Work out the finished part from the listing and answer in its coordinate system (mm). A direction names the side the tool comes from. Coordinates: 2 decimals unless noted, no trailing zeros. Order: outer loops, then holes, each group sorted by start corner. A loop starts at its lowest first (then second) coordinate and runs counter-clockwise, first axis right, second up.
```python
from build123d import *

# Parameters (mm, degrees)
SKETCH1_R           = 133
BOSS_EXTRUDE1_DEPTH = 53.5
SKETCH2_R           = 125
BOSS_EXTRUDE2_DEPTH = 51
SKETCH3_R           = 100
BOSS_EXTRUDE3_DEPTH = 5
SKETCH4_R           = 106
BOSS_EXTRUDE4_DEPTH = 12
SKETCH5_R           = 60
BOSS_EXTRUDE5_DEPTH = 11
SKETCH6_R           = 35
CUT_EXTRUDE1_DEPTH  = 231.074444474


with BuildPart() as part:
    # Sketch1 → Boss-Extrude1 (new body)
    with BuildSketch(Plane(origin=(0, 0, 0), x_dir=(1, 0, 0), z_dir=(0, 1, 0))):
        with Locations(Location((0, 0, 0), (0, 0, 270))):
            Circle(SKETCH1_R)
    extrude(amount=BOSS_EXTRUDE1_DEPTH)

    # Sketch2 → Boss-Extrude2 (add)
    with BuildSketch(Plane(origin=(0, 53.5, 0), x_dir=(1, 0, 0), z_dir=(0, 1, 0))):
        with Locations(Location((0, 0, 0), (0, 0, 270))):
            Circle(SKETCH2_R)
    extrude(amount=BOSS_EXTRUDE2_DEPTH)

    # Sketch3 → Boss-Extrude3 (add)
    with BuildSketch(Plane(origin=(0, 104.5, 0), x_dir=(1, 0, 0), z_dir=(0, 1, 0))):
        with Locations(Location((0, 0, 0), (0, 0, 270))):
            Circle(SKETCH3_R)
    extrude(amount=BOSS_EXTRUDE3_DEPTH)

    # Sketch4 → Boss-Extrude4 (add)
    with BuildSketch(Plane.XZ):
        with Locations(Location((0, 0, 0), (0, 0, 270))):
            Circle(SKETCH4_R)
    extrude(amount=BOSS_EXTRUDE4_DEPTH)

    # Sketch5 → Boss-Extrude5 (add)
    with BuildSketch(Plane.XZ.offset(12)):
        with Locations(Location((0, 0, 0), (0, 0, 270))):
            Circle(SKETCH5_R)
    extrude(amount=BOSS_EXTRUDE5_DEPTH)

    # Sketch6 → Cut-Extrude1 (cut, through all)
    with BuildSketch(Plane.XZ.offset(23)):
        with Locations(Location((0, 0, 0), (0, 0, 270))):
            Circle(SKETCH6_R)
    extrude(amount=-CUT_EXTRUDE1_DEPTH, mode=Mode.SUBTRACT)


solid = part.part
```
1. The part is cut by section A-A (z = 0). Determine the outline of the cut face in (x, y).
2. Consider probe 1 along X at (y, z) = (67, 0); probe 2 along X at (y, z) = (61.5, -3); probe 3 along Y at (x, z) = (-95.5, 70). Determine where each line is inside the solid, lowest interval first.
3. The part is cut by section C-C (y = 64). Determine the outline of the cut face in (x, z).
4. Flat-ended cylindrical pins translate along their axes: pin 1 (1.5 mm diameter, centred on y = 59.5, z = -82, fed in from +X); pin 2 (6 mm diameter, centred on x = 97.5, z = -75.5, fed in from -Y); pin 3 (1.5 mm diameter, centred on y = 27.5, z = -101.5, fed in from +X). Find the tip coordinate at first contact, or state that the pin passes through.
5. The part is cut by section B-B (x = 0). Determine the outline of the cut face in (y, z).
6. The part is cut by section D-D (z = 49.5). Determine the outline of the cut face in (x, y), plus the area to 3 significant figures.
7. For faces 1 (the flat face through (-46, -12, -46)), 2 (the flat face through (-43, 109.5, -1)), 3 (the flat face through (84, 104.5, -56)), determine the directions among +Z, -Z, +X, -X, +Y, -Y from which every point of the face is accessible in a straight line to the end or side of a thin tool.
Worked out:
1. outline: (-133, 0) - (-106, 0) - (-106, -12) - (-60, -12) - (-60, -23) - (-35, -23) - (-35, 109.5) - (-100, 109.5) - (-100, 104.5) - (-125, 104.5) - (-125, 53.5) - (-133, 53.5) - close; (35, -23) - (60, -23) - (60, -12) - (106, -12) - (106, 0) - (133, 0) - (133, 53.5) - (125, 53.5) - (125, 104.5) - (100, 104.5) - (100, 109.5) - (35, 109.5) - close
2. probe 1: x = -125 to -35, 35 to 125
2. probe 2: x = -124.96 to -34.87, 34.87 to 124.96
2. probe 3: y = 0 to 104.5
3. outline: circle Ø250 at (0, 0); hole circle Ø70 at (0, 0)
4. pin 1: stops at x = 94.99
4. pin 2: stops at y = 0
4. pin 3: stops at x = 86.82
5. outline: (-23, -60) - (-12, -60) - (-12, -106) - (0, -106) - (0, -133) - (53.5, -133) - (53.5, -125) - (104.5, -125) - (104.5, -100) - (109.5, -100) - (109.5, -35) - (-23, -35) - close; (-23, 35) - (109.5, 35) - (109.5, 100) - (104.5, 100) - (104.5, 125) - (53.5, 125) - (53.5, 133) - (0, 133) - (0, 106) - (-12, 106) - (-12, 60) - (-23, 60) - close
6. outline: (-123.45, 0) - (-93.73, 0) - (-93.73, -12) - (-33.91, -12) - (-33.91, -23) - (33.91, -23) - (33.91, -12) - (93.73, -12) - (93.73, 0) - (123.45, 0) - (123.45, 53.5) - (114.78, 53.5) - (114.78, 104.5) - (86.89, 104.5) - (86.89, 109.5) - (-86.89, 109.5) - (-86.89, 104.5) - (-114.78, 104.5) - (-114.78, 53.5) - (-123.45, 53.5) - close
6. area: 28,800 mm2
7. face 1: -Y
7. face 2: +Z, -Z, +X, -X, +Y
7. face 3: +Y
